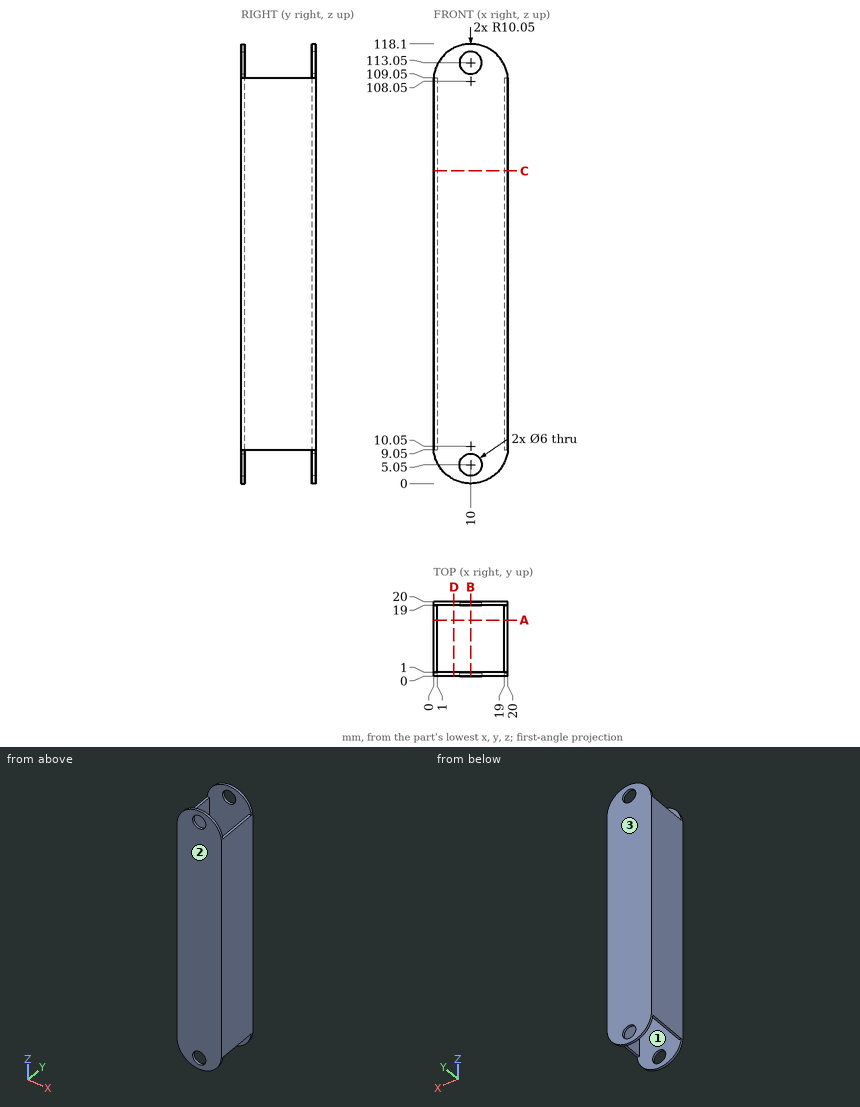
Geometry: see drawing. Coordinates: mm, zero at the bounding-box minimum. Round coordinates to 2 decimals unless told otherwise and drop trailing zeros. Order: outer loops, then holes, each group sorted by start corner. A loop starts at its lowest first (then second) coordinate and runs counter-clockwise, first axis right, second up. Notation, with made-up numbers: (-13.5, 24.5) -> (-3.5, 24.5) arc R23 ccw to (-3.5, 41.5) -> close; hole circle Ø9 at (69.5, -0.5). An arc over 180 degrees is marked (long way). Answer as CSV lines item,"result".
Item 1: Section B-B, the plane x = 10. Return loops of the section in (y, z).
A:
outline,"(0, 0) -> (1, 0) -> (1, 2.05) -> (0, 2.05) -> close; (0, 8.05) -> (1, 8.05) -> (1, 110.05) -> (0, 110.05) -> close; (0, 116.05) -> (1, 116.05) -> (1, 118.1) -> (0, 118.1) -> close; (19, 0) -> (20, 0) -> (20, 2.05) -> (19, 2.05) -> close; (19, 8.05) -> (20, 8.05) -> (20, 110.05) -> (19, 110.05) -> close; (19, 116.05) -> (20, 116.05) -> (20, 118.1) -> (19, 118.1) -> close"
Item 2: Pin query (flat end, axial travel): pin 1 Ø6 at (x, z) = (11, 63) entering from -Y; pin 2 Ø5 at (x, y) = (6.5, 4.5) entering from +Z; pin 3 Ø0.8 at (x, y) = (0.5, 12) entering from +Z; pin 4 Ø1.1 at (x, y) = (19.5, 13) entering from -Z. Return the tip coordinate at first contact, or that it passes through.
A:
pin 1,"y = 0"
pin 2,"through"
pin 3,"z = 109.05"
pin 4,"z = 9.05"
Item 3: Section D-D, the plane x = 5.5. Return loops of the section in (y, z).
A:
outline,"(0, 1.06) -> (1, 1.06) -> (1, 117.04) -> (0, 117.04) -> close; (19, 1.06) -> (20, 1.06) -> (20, 117.04) -> (19, 117.04) -> close"
Item 4: Section A-A, the plane y = 15. Return loops of the section in (x, z).
A:
outline,"(0, 9.05) -> (1, 9.05) -> (1, 109.05) -> (0, 109.05) -> close; (19, 9.05) -> (20, 9.05) -> (20, 109.05) -> (19, 109.05) -> close"
Item 5: Pull-direction query (Y, two-part tool) for the marked faces 1, 2 and 3; classes: pulls with the +Y half, pulls with the -Y half, needs draft (parallel to the pull), parting line crosses it, or undercut.
A:
face 1,"undercut"
face 2,"pulls with the -Y half"
face 3,"pulls with the +Y half"
Item 6: Line query: L1, parallel to Z at x = 10, y = 19.7; L2, parallel to Y at x = 7, z = 61.5. Output: solid intervals per line, ascending.
A:
L1,"0 to 2.05, 8.05 to 110.05, 116.05 to 118.1"
L2,"0 to 1, 19 to 20"
Item 7: Section C-C, the plane z = 84. Return loops of the section in (x, y).
A:
outline,"(0, 0) -> (20, 0) -> (20, 20) -> (0, 20) -> close; hole (1, 1) -> (19, 1) -> (19, 19) -> (1, 19) -> close"
